Autodesk Fusion 360 part; units mm, degrees
sketch "Sketch1" plane through (0, 0, 0) normal (0, 1, 0) x (1, 0, 0)
  line L0 (0, 0) -> (-25, 0)
  line L1 (-25, 0) -> (-25, -5)
  line L2 (-25, -5) -> (5, -5)
  line L3 (0, 0) -> (0, 10)
  line L4 (0, 10) -> (5, 10)
  line L5 (5, 10) -> (5, -5)
  line L6 (-25, 0) -> (-245, 0)
  line L7 (-245, 0) -> (-245, -5)
  line L8 (-245, -5) -> (-25, -5)
  line L9 (-25, 0) -> (-140, 0)
  line L10 (-140, 0) -> (-140, 27.0089)
  line L11 (-270, 10) -> (-275, 10)
  line L12 (-270, 0) -> (-270, 10)
  line L13 (-275, 10) -> (-275, -5)
  line L14 (-270, 0) -> (-245, 0)
  line L15 (-245, -5) -> (-275, -5)
  line L16 (-245, 0) -> (-245, -5)
  point P0 (-270, 0)
  dimension "d1" = 25
  dimension "d2" = 5
  dimension "d3" = 30
  dimension "d4" = 10
  dimension "d5" = 5
  dimension "d6" = 220
  dimension "d7" = 5
  dimension "d8" = 115
extrude "Extrude1" add sketch "Sketch1" along normal blind 10
extrude "Extrude2" add sketch "Sketch1" along normal blind 20 contours L0 L1 L2 L3 L4 L5 | L7 L11 L12 L13 L14 L15 L16
sketch "Sketch2" plane through (5, 0, 0) normal (1, 0, 0) x (0, 0, -1)
  line L0 (-5, 0) -> (10, 0)
  line L1 (10, 0) -> (10, 20)
  line L2 (10, 20) -> (-5, 20)
  line L3 (-5, 20) -> (-5, 0)
sketch "Sketch3" plane through (0, 0, 0) normal (-1, 0, 0) x (0, 0, 1)
  line L0 (-10, 0) -> (0, 0)
  line L1 (0, 0) -> (0, 20)
  line L2 (0, 20) -> (-10, 20)
  line L3 (-10, 20) -> (-10, 0)
  line L4 (-10, 0) -> (-5, 0)
  line L5 (-5, 0) -> (-5, 10)
  circle A0 centre (-5, 10) radius 2.5
  dimension "d13" = 5
  dimension "d14" = 10
  dimension "d15" = 5
extrude "Extrude3" cut sketch "Sketch3" along normal mid plane 662 contours A0
chamfer "Chamfer1" distance 5 angle 45 4 edges at (2.5, 20, -10) (2.5, 0, -10) (-272.5, 20, -10) (-272.5, 0, -10)
The listing builds one solid part. Answer for the finished solid, in the listing's coordinates (mm). A direction names the side the tool comes from. Give positions to 0.01 mm unless a question says otherwise; leave off trailing zeros. Write each loop counter-clockwise with the first axis right and the second up, starting at its lowest first coordinate (ties: lowest second). Pieces come first, ordered by that corner, then holes. Notation, with made-up numbers: (42.5, 64.5) -> (88.5, 64.5) arc R29 cw to (88.5, 93.5) -> close; hole circle Ø5 at (45.5, -4.5). An arc over 180 degrees is marked (long way). Write item = value, one per line. Start each with the question number.
1) Determine the mould class of faces 1 (the face through (0, 7.6, -3.8)), 2 (the face through (-275, 10, -1)), 3 (the face through (-264, 20, 2)) for opening direction X: +X half, -X half, draft (parallel to the pull), parting line (faces both ways), or undercut.
2) Which of the six approach directions +Z, -Z, +X, -X, +Y, -Y give full straight-line access (tool end or side, diameter ignored) to faces 4 (the face through (-133, 8, 0)), 5 (the face through (-245, 15, 2)), 6 (the face through (2, 3, -8))?
3) The part is cut by section A-A, the plane x = -121. Determine the outline of the cut face in (y, z).
4) Each of these flat-tipped pins is pushed along its axis until it touches: pin 1 (6 mm diameter, centred on x = -126, y = 2, fed in from -Z); pin 2 (5.5 mm diameter, centred on x = -134.5, z = 3, fed in from +Y); pin 3 (3 mm diameter, centred on y = 10, z = -5, fed in from +X). Where does it stop, or does it pass through?
5) Straight lines are drawn through the part: line 1 along X through (y, z) = (13.5, 2.25); line 2 along Y through (x, z) = (3.6, -5); line 3 along X through (y, z) = (8.25, -3). For each, find the intervals that lie inside material, in ascending order.
Solutions:
q1.face_1 = undercut
q1.face_2 = -X half
q1.face_3 = draft
q2.face_4 = -Z, +Y, -Y
q2.face_5 = +Z, -Z, +Y
q2.face_6 = -Z, +X, -X, -Y
q3.outline = (0, 0) -> (10, 0) -> (10, 5) -> (0, 5) -> close
q4.pin_1 = 0
q4.pin_2 = 10
q4.pin_3 = through
q5.line_1 = -275 to -245, -25 to 5
q5.line_2 = 0 to 7.5, 12.5 to 20
q5.line_3 = -275 to -270, 0 to 5
